from build123d import *

# Parameters (mm, degrees)
SKETCH1_R           = 3.3
BOSS_EXTRUDE1_DEPTH = 2.4
FILLET1_R           = 0.8
SKETCH2_R           = 2
BOSS_EXTRUDE2_DEPTH = 7
CUT_EXTRUDE1_DEPTH  = 2
CUT_EXTRUDE1_DRAFT  = -6
FILLET2_R           = 0.1
LPATTERN1_COUNT     = 17
LPATTERN1_PITCH     = 0.4


with BuildPart() as part:
    # Sketch1 → Boss-Extrude1 (new body)
    with BuildSketch(Plane.XY):
        Circle(SKETCH1_R)
    extrude(amount=BOSS_EXTRUDE1_DEPTH)

    # Fillet1
    fillet1_edges = [part.edges().sort_by_distance(p)[0] for p in [
        (-3.3, 0, 2.4),
    ]]
    fillet(fillet1_edges, radius=FILLET1_R)

    # Sketch2 → Boss-Extrude2 (add)
    with BuildSketch(Plane(origin=(0, 0, 0), x_dir=(-1, 0, 0), z_dir=(0, 0, -1))):
        with Locations(Location((0, 0, 0), (0, 0, 180))):
            Circle(SKETCH2_R)
    extrude(amount=BOSS_EXTRUDE2_DEPTH)


with BuildPart() as cut_extrude1_tool:
    # Sketch4 → Cut-Extrude1 (with draft: the straight prism first)
    with BuildSketch(Plane.XY.offset(2.4)):
        with BuildLine():
            Line((-0.4, -2), (0.4, -2))
            Line((0.4, -2), (0.4, -0.9))
            ThreePointArc((0.4, -0.9), (0.546446609, -0.546446609), (0.9, -0.4))
            Line((0.9, -0.4), (2, -0.4))
            Line((2, -0.4), (2, 0.4))
            Line((2, 0.4), (0.9, 0.4))
            ThreePointArc((0.9, 0.4), (0.546446609, 0.546446609), (0.4, 0.9))
            Line((0.4, 0.9), (0.4, 2))
            Line((0.4, 2), (-0.4, 2))
            Line((-0.4, 2), (-0.4, 0.9))
            ThreePointArc((-0.4, 0.9), (-0.546446609, 0.546446609), (-0.9, 0.4))
            Line((-0.9, 0.4), (-2, 0.4))
            Line((-2, 0.4), (-2, -0.4))
            Line((-2, -0.4), (-0.9, -0.4))
            ThreePointArc((-0.9, -0.4), (-0.546446609, -0.546446609), (-0.4, -0.9))
            Line((-0.4, -0.9), (-0.4, -2))
        make_face()
    extrude(amount=-CUT_EXTRUDE1_DEPTH)
    # Cut-Extrude1: the draft: its side faces are tilted about the plane it starts from
    cut_extrude1_sides = [cut_extrude1_tool.faces().sort_by_distance(p)[0] for p in [
        (-0.4, -1.45, 1.4),
        (0, -2, 1.4),
        (0.4, -1.45, 1.4),
        (0.546446609, -0.546446609, 1.4),
        (1.45, -0.4, 1.4),
        (2, 0, 1.4),
        (1.45, 0.4, 1.4),
        (0.546446609, 0.546446609, 1.4),
        (0.4, 1.45, 1.4),
        (0, 2, 1.4),
        (-0.4, 1.45, 1.4),
        (-0.546446609, 0.546446609, 1.4),
        (-1.45, 0.4, 1.4),
        (-2, 0, 1.4),
        (-1.45, -0.4, 1.4),
        (-0.546446609, -0.546446609, 1.4),
    ]]
    draft(cut_extrude1_sides, Plane.XY.offset(2.4), CUT_EXTRUDE1_DRAFT)


with BuildPart() as part_1:
    add(part.part)

    # Cut-Extrude1: cut by cut_extrude1_tool
    add(cut_extrude1_tool.part, mode=Mode.SUBTRACT)

    # Fillet2
    fillet2_edges = [part_1.edges().sort_by_distance(p)[0] for p in [
        (0.4, 1.45, 2.4),
        (0, 2, 2.4),
        (-0.4, 1.45, 2.4),
        (-0.546446609, 0.546446609, 2.4),
        (-1.45, 0.4, 2.4),
        (-2, 0, 2.4),
        (-1.45, -0.4, 2.4),
        (-0.546446609, -0.546446609, 2.4),
        (-0.4, -1.45, 2.4),
        (0, -2, 2.4),
        (0.4, -1.45, 2.4),
        (0.546446609, -0.546446609, 2.4),
        (1.45, -0.4, 2.4),
        (2, 0, 2.4),
        (1.45, 0.4, 2.4),
        (0.546446609, 0.546446609, 2.4),
    ]]
    fillet(fillet2_edges, radius=FILLET2_R)

    # Sketch5 → Cut-Revolve1 (revolve, cut)
    with BuildSketch(Plane(origin=(0, 0, 0), x_dir=(0, 0, -1), z_dir=(1, 0, 0)), mode=Mode.PRIVATE) as cut_revolve1_sk:
        Polygon((7, 1.7), (7.2, 2.01), (6.8, 2.01), align=None)
    cut_revolve1 = revolve(cut_revolve1_sk.sketch.rotate(Axis((0, 0, 0), (0, 0, -1)), 90), axis=Axis((0, 0, 0), (0, 0, -1)), mode=Mode.SUBTRACT)

    # LPattern1: Cut-Revolve1 ×17
    with Locations(*[(0, 0, i * LPATTERN1_PITCH) for i in range(1, LPATTERN1_COUNT)]):
        add(cut_revolve1, mode=Mode.SUBTRACT)


solid = part_1.part
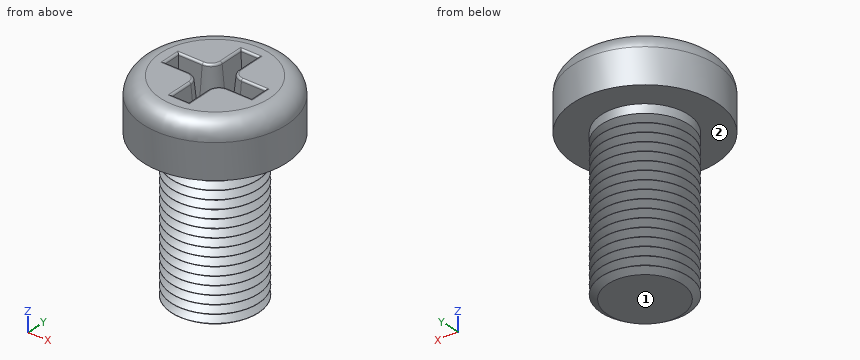
Model file for the job. Use its own axes, mm. Face numbers are marked on the shaded views. A direction names the side the tool comes from. Coordinates: 2 decimals unless noted, no trailing zeros. Write each loop counter-clockwise with the first axis right and the second up, starting at its lowest first coordinate (ties: lowest second). Pieces come first, ordered by that corner, then holes. Notation, with made-up numbers: (34.25, -0.75) -> (89.25, -0.75) arc R17 cw to (89.25, 31.25) -> close; hole circle Ø3 at (0.5, 83.5). An arc over 180 degrees is marked (long way). One line per item, written item: value. Start each with the question number.
1) Which spindle directions (+Z, -Z, +X, -X, +Y, -Y) get a long thin tool onto all of the face, cutting with end or side? Do the marked faces 1 and 2. Say none if no direction does.
2) Flat gauge pin, fed straight in: pin 1 Ø1.1 at (x, y) = (0.5, 0.5) entering from +Z. Where does the tip first touch, or does it go through?
3) Probe probe 1 along Z at (x, y) = (1.5, 1.75); probe 2 along Y at (x, z) = (0, 0.75); probe 3 along X at (y, z) = (3, 0.25). List the from-to ranges inside material, lowest first.
4) Slice it at A-A on z = 1.25. Write the cut outline in (x, y), then the cut area to 3 significant figures.
Answers follow:
1. face 1: -Z, +X, -X, +Y, -Y
1. face 2: -Z
2. pin 1: z = 2.4
3. probe 1: 0 to 2.4
3. probe 2: -3.3 to -1.83, 1.83 to 3.3
3. probe 3: -1.37 to 1.37
4. outline: circle Ø6.6 at (0, 0); hole (-1.88, -0.28) -> (-0.9, -0.28) arc R0.62 cw to (-0.28, -0.9) -> (-0.28, -1.88) -> (0.28, -1.88) -> (0.28, -0.9) arc R0.62 cw to (0.9, -0.28) -> (1.88, -0.28) -> (1.88, 0.28) -> (0.9, 0.28) arc R0.62 cw to (0.28, 0.9) -> (0.28, 1.88) -> (-0.28, 1.88) -> (-0.28, 0.9) arc R0.62 cw to (-0.9, 0.28) -> (-1.88, 0.28) -> close
4. area: 30.0 mm2
